Read the model definition and answer for the solid it produces. Units are mm, in the model's axes. Coordinates: 2 decimals unless noted, no trailing zeros. Loops run counter-clockwise (first coordinate to the right, second up) from the corner with the lowest first, then second, coordinate; pieces in that order, holes last. Notation, with made-up numbers: M 53,-15 L 66,-15 A26 cw 66,11 Z; hole C 42.25,-9.5 d10. An arc over 180 degrees is marked long. One line per item, written item: value. Start each with the question number.
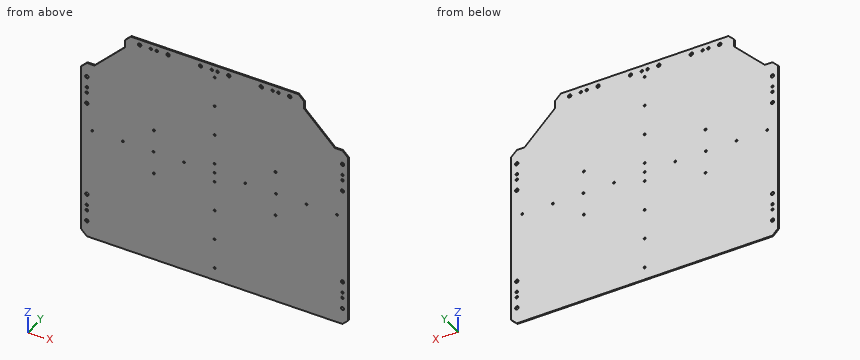
Autodesk Inventor part; units mm, degrees
ref_plane "YZ Plane" through (0, 0, 0) normal (1, 0, 0) x (0, 1, 0)
ref_plane "XZ Plane" through (0, 0, 0) normal (0, 1, 0) x (-1, 0, 0)
ref_plane "XY Plane" through (0, 0, 0) normal (0, 0, 1) x (1, 0, 0)
sketch "Skizze1" plane through (0, 0, 0) normal (0, 1, 0) x (-1, 0, 0)
  line L0 (0, 0) -> (-698, 0)
  line L1 (-698, 0) -> (-698, 597)
  line L2 (-698, 597) -> (0, 597)
  line L3 (0, 597) -> (0, 0)
  line L4 (-349, 0) -> (-349, 597) construction
  line L5 (0, 298.5) -> (-698, 298.5) construction
  line L6 (-190, 0) -> (-190, 597) construction
  line L7 (-508, 0) -> (-508, 597) construction
  line L8 (-698, 407) -> (0, 407) construction
  line L9 (0, 80) -> (-698, 80) construction
  line L10 (-683, 582) -> (-683, 15) construction
  line L11 (-683, 15) -> (-15, 15) construction
  line L12 (-15, 15) -> (-15, 582) construction
  line L13 (-15, 582) -> (-683, 582) construction
  line L14 (-23, 362) -> (-7, 362) construction
  line L15 (-7, 362) -> (-7, 452) construction
  line L16 (-7, 452) -> (-23, 452) construction
  line L17 (-23, 452) -> (-23, 362) construction
  line L18 (-23, 362) -> (-7, 452) construction
  line L19 (-7, 362) -> (-23, 452) construction
  line L20 (-145, 590) -> (-235, 590) construction
  line L21 (-235, 590) -> (-235, 574) construction
  line L22 (-235, 574) -> (-145, 574) construction
  line L23 (-145, 574) -> (-145, 590) construction
  line L24 (-145, 590) -> (-235, 574) construction
  line L25 (-235, 590) -> (-145, 574) construction
  line L26 (-304, 590) -> (-394, 590) construction
  line L27 (-394, 590) -> (-394, 574) construction
  line L28 (-394, 574) -> (-304, 574) construction
  line L29 (-304, 574) -> (-304, 590) construction
  line L30 (-304, 590) -> (-394, 574) construction
  line L31 (-394, 590) -> (-304, 574) construction
  circle A0 centre (-15, 399.5) radius 3.25
  circle A1 centre (-15, 370) radius 4.5
  circle A2 centre (-15, 414.5) radius 3.25
  circle A3 centre (-15, 444) radius 4.5
  circle A4 centre (-182.5, 582) radius 3.25
  circle A5 centre (-153, 582) radius 4.5
  circle A6 centre (-312, 582) radius 4.5
  circle A7 centre (-341.5, 582) radius 3.25
  circle A8 centre (-197.5, 582) radius 3.25
  circle A9 centre (-227, 582) radius 4.5
  circle A10 centre (-386, 582) radius 4.5
  circle A11 centre (-356.5, 582) radius 3.25
  circle A12 centre (-683, 399.5) radius 3.25
  circle A13 centre (-683, 370) radius 4.5
  circle A14 centre (-683, 444) radius 4.5
  circle A15 centre (-683, 414.5) radius 3.25
  circle A16 centre (-515.5, 582) radius 3.25
  circle A17 centre (-545, 582) radius 4.5
  circle A18 centre (-500.5, 582) radius 3.25
  circle A19 centre (-471, 582) radius 4.5
  circle A20 centre (-15, 43) radius 4.5
  circle A21 centre (-15, 72.5) radius 3.25
  circle A22 centre (-190, 238.5) radius 2.75
  circle A23 centre (-190, 358.5) radius 2.75
  circle A24 centre (-508, 238.5) radius 2.75
  circle A25 centre (-508, 358.5) radius 2.75
  circle A26 centre (-15, 117) radius 4.5
  circle A27 centre (-15, 87.5) radius 3.25
  circle A28 centre (-683, 43) radius 4.5
  circle A29 centre (-683, 72.5) radius 3.25
  circle A30 centre (-683, 87.5) radius 3.25
  circle A31 centre (-683, 117) radius 4.5
  line L32 (0, 482) -> (-35, 482)
  line L33 (-35, 482) -> (-115, 562)
  line L34 (-115, 562) -> (-115, 597)
  line L35 (-698, 482) -> (-663, 482)
  line L36 (-663, 482) -> (-583, 562)
  line L37 (-583, 562) -> (-583, 597)
  point P0 (-15, 407)
  point P1 (-190, 582)
  point P2 (-349, 582)
  point P3 (-190, 298.5)
  dimension "d0" = 698
  dimension "d1" = 597
  dimension "d2" = 190
  dimension "d3" = 80
  dimension "d4" = 190
  dimension "d5" = 190
  dimension "d6" = 15
  dimension "d7" = 16
  dimension "d8" = 90
  dimension "d9" = 90
  dimension "d10" = 16
  dimension "d11" = 90
  dimension "d12" = 16
  dimension "d13" = 6.5
  dimension "d14" = 7.5
  dimension "d15" = 9
  dimension "d16" = 37
  dimension "d17" = 6.5
  dimension "d18" = 9
  dimension "d19" = 7.5
  dimension "d20" = 37
  dimension "d21" = 6.5
  dimension "d22" = 9
  dimension "d23" = 7.5
  dimension "d24" = 37
  dimension "d30" = 5.5
  dimension "d34" = 6.5
  dimension "d35" = 9
  dimension "d36" = 7.5
  dimension "d37" = 37
  dimension "d80" = 115
  dimension "d81" = 115
  dimension "d82" = 45
  dimension "d83" = 35
extrude "Ex-Platte" add sketch "Skizze1" along normal blind 3 contours L0 L1 L35 L36 L37 L2 L34 L33 L32 L3
chamfer "Fase-15mm" distance 15 angle 45 6 edges at (698, 1.5, 0) (0, 1.5, 0) (0, 1.5, 482) (115, 1.5, 597) (583, 1.5, 597) (698, 1.5, 482)
sketch "Profil-Verstärkung" plane through (0, 0, 0) normal (0, 1, 0) x (-1, 0, 0)
  line L0 (-683, 0) -> (-15, 0)
  line L1 (0, 15) -> (0, 482)
  line L2 (-115, 597) -> (-583, 597)
  line L3 (-698, 482) -> (-698, 15)
  line L4 (0, 298.5) -> (-698, 298.5) construction
  circle A0 centre (-15, 117) radius 4.5
  circle A1 centre (-15, 370) radius 4.5
  circle A2 centre (-190, 358.5) radius 2.75
  circle A3 centre (-190, 238.5) radius 2.75
  circle A4 centre (-227, 582) radius 4.5
  circle A5 centre (-312, 582) radius 4.5
  line L5 (-349, 0) -> (-349, 597) construction
  circle A6 centre (-349, 298.5) radius 2.5
  circle A7 centre (-429, 298.5) radius 2.5
  circle A8 centre (-509, 298.5) radius 2.5
  circle A9 centre (-589, 298.5) radius 2.5
  circle A10 centre (-669, 298.5) radius 2.5
  circle A11 centre (-349, 323.5) radius 2.5
  circle A12 centre (-349, 403.5) radius 2.5
  circle A13 centre (-349, 483.5) radius 2.5
  circle A14 centre (-349, 563.5) radius 2.5
  circle A15 centre (-269, 298.5) radius 2.5
  circle A16 centre (-189, 298.5) radius 2.5
  circle A17 centre (-109, 298.5) radius 2.5
  circle A18 centre (-29, 298.5) radius 2.5
  circle A19 centre (-349, 273.5) radius 2.5
  circle A20 centre (-349, 193.5) radius 2.5
  circle A21 centre (-349, 113.5) radius 2.5
  circle A22 centre (-349, 33.5) radius 2.5
  point P0 (0, 0)
  point P1 (0, 582)
  point P2 (-15, 597)
  point P3 (-683, 597)
  point P4 (-698, 582)
  dimension "d38" = 698
  dimension "d40" = 121.5
  dimension "d42" = 11.5
  dimension "d61" = 5
  dimension "d64" = 80
  dimension "d69" = 5
  dimension "d70" = 25
  dimension "d73" = 80
extrude "Ex-ProfilBohrungen" cut sketch "Profil-Verstärkung" along normal up to surface (3 mm away) contours A6 | A7 | A8 | A9 | A10 | A11 | A12 | A13 | A14 | A15 | A16 | A17 | A18 | A19 | A20 | A21 | A22
equation "\"d5\" = d4"
equation "\"d17\" = d13"
equation "\"d18\" = d15"
equation "\"d19\" = d14"
equation "\"d20\" = d16"
equation "\"d21\" = d13"
equation "\"d22\" = d15"
equation "\"d23\" = d14"
equation "\"d24\" = d16"
equation "\"d34\" = d13"
equation "\"d35\" = d15"
equation "\"d36\" = d14"
equation "\"d37\" = d16"
equation "\"d81\" = d80"
equation "\"d69\" = d61"
properties part number "enc-SidePanel Unten 575x708"
1) Section A-A (y = 1.75) is taken. Count the separate pieces of the cut face and the enclosed holes in it, then the cut area to 3 significant figures.
2) Section B-B (x = 64) is taken. Determine the outline of the cut face in (y, z), then the cut area to 3 significant figures.
3) Consider line 1 along X through (y, z) = (0.7, 34); line 2 along X through (y, z) = (1.6, 399.5); line 3 along Z through (x, y) = (153, 1.4). Determine where each line is inside the solid, lowest interval first.
Results found:
1. separate pieces: 1
1. enclosed holes: 49
1. area: 394,000 mm²
2. outline: M 0,0 L 3,0 L 3,511 L 0,511 Z
2. area: 1,530 mm²
3. line 1: x = 0 to 346.55, 351.45 to 698
3. line 2: x = 0 to 11.75, 18.25 to 679.75, 686.25 to 698
3. line 3: z = 0 to 577.5, 586.5 to 597
